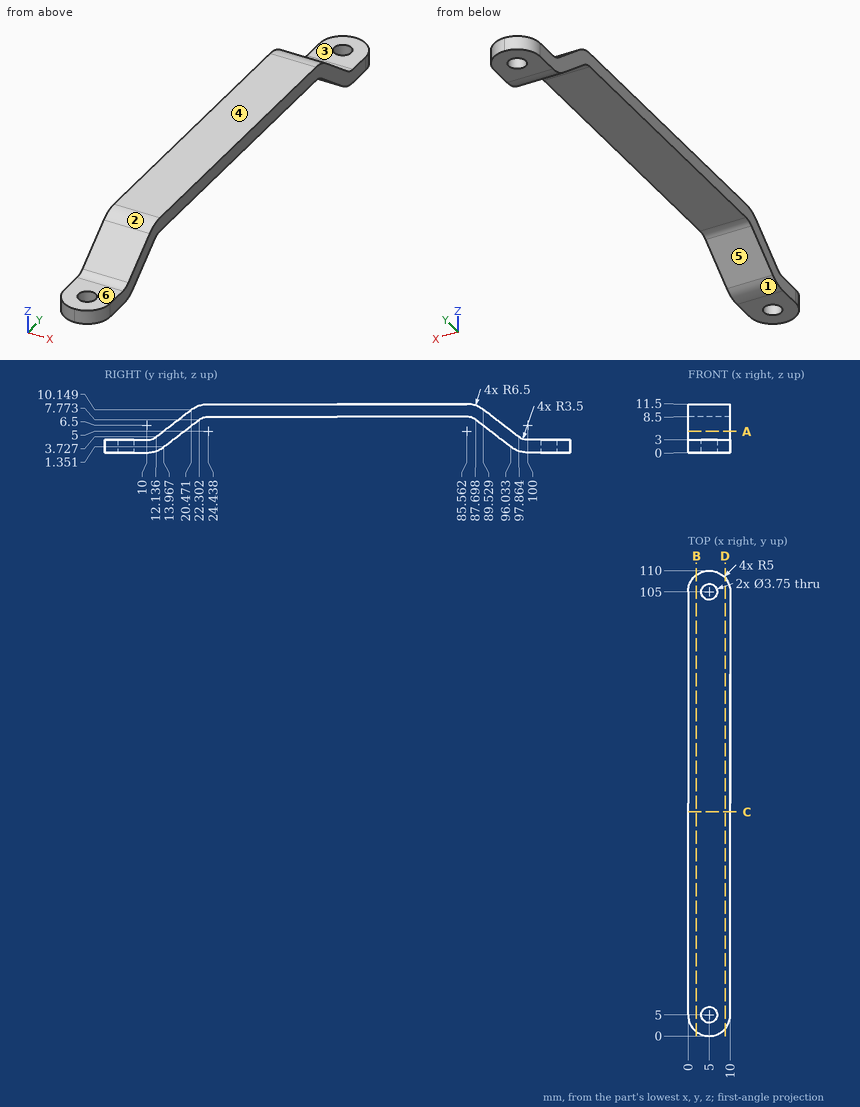
Check sheet for the drawn part. Datum: minimum x, y, z corner. Units: mm. A direction names the side the tool comes from. Round coordinates to 2 decimals unless told otherwise and drop trailing zeros. Order: outer loops, then holes, each group sorted by start corner. A loop starts at its lowest first (then second) coordinate and runs counter-clockwise, first axis right, second up. Notation, with made-up numbers: (79, 63.25) - (102, 63.25) arc R26 ccw to (102, 92.25) - close; hole circle Ø4 at (40, 0.5). An arc over 180 degrees is marked (long way). Use a Markdown table: item, result. Add a question column.
(1) Tool access check on the marked faces 4, 5 and 6. Record the directions out of +Z, -Z, +X, -X, +Y, -Y that give a thin tool (end or side, any length) a straight path to the whole face; none if there is none.
(2) Release check for a two-part mould opening along Y. For the marked faces 1, 2 and 3 record: pulls with the +Y half, pulls with the -Y half, needs draft (parallel to the pull), parting line crosses it, or undercut.
(3) Sectioned sample at C-C, the plane y = 53. Enter the section's corners in (x, z).
(4) Sectioned sample at D-D, the plane x = 8.75. Enter the section's corners in (y, z), and give its area (3 significant figures).
(5) Depth check by flat-ended pin: pin 1 (3 mm diameter, centred on x = 6, z = 10.5, fed in from +Y); pin 2 (5 mm diameter, centred on x = 6, y = 41, fed in from -Z); pin 3 (3.5 mm diameter, centred on x = 5, y = 105, fed in from +Z); pin 4 (5 mm diameter, centred on x = 7.5, y = 5, fed in from +Z). Enter the tip coordinate at first touch or a pass-through.
(6) Sectioned sample at A-A, the plane z = 5. Enter the section's corners in (x, y).
(7) Sectioned sample at B-B, the plane x = 2. Enter the section's corners in (y, z).
(8) Material ranges on line 1 along Y through (x, z) = (5, 1.75) (1 decimal); line 2 along Y through (x, z) = (5, 1.6) (1 decimal); line 3 along X through (y, z) = (105, 1.4) (1 decimal), recorded low to high. Write a range as [from, to].
Answers below:
| question | item | result |
|---|---|---|
| 1 | face 4 | +Z, +X, -X, +Y, -Y |
| 1 | face 5 | -Z, +X, -X |
| 1 | face 6 | +Z, +X, -X, -Y |
| 2 | face 1 | undercut |
| 2 | face 2 | pulls with the -Y half |
| 2 | face 3 | needs draft |
| 3 | outline | (0, 8.5) - (10, 8.5) - (10, 11.5) - (0, 11.5) - close |
| 4 | outline | (1.69, 0) - (10, 0) arc R6.5 ccw to (13.97, 1.35) - (22.3, 7.77) arc R3.5 cw to (24.44, 8.5) - (85.56, 8.5) arc R3.5 cw to (87.7, 7.77) - (96.03, 1.35) arc R6.5 ccw to (100, 0) - (108.31, 0) - (108.31, 3) - (100, 3) arc R3.5 cw to (97.86, 3.73) - (89.53, 10.15) arc R6.5 ccw to (85.56, 11.5) - (24.44, 11.5) arc R6.5 ccw to (20.47, 10.15) - (12.14, 3.73) arc R3.5 cw to (10, 3) - (1.69, 3) - close |
| 4 | area | 336 mm² |
| 5 | pin 1 | y = 91.02 |
| 5 | pin 2 | z = 8.5 |
| 5 | pin 3 | through |
| 5 | pin 4 | z = 3 |
| 6 | outline | (0, 13.79) - (10, 13.79) - (10, 18.7) - (0, 18.7) - close; (0, 91.3) - (10, 91.3) - (10, 96.21) - (0, 96.21) - close |
| 7 | outline | (1, 0) - (10, 0) arc R6.5 ccw to (13.97, 1.35) - (22.3, 7.77) arc R3.5 cw to (24.44, 8.5) - (85.56, 8.5) arc R3.5 cw to (87.7, 7.77) - (96.03, 1.35) arc R6.5 ccw to (100, 0) - (109, 0) - (109, 3) - (100, 3) arc R3.5 cw to (97.86, 3.73) - (89.53, 10.15) arc R6.5 ccw to (85.56, 11.5) - (24.44, 11.5) arc R6.5 ccw to (20.47, 10.15) - (12.14, 3.73) arc R3.5 cw to (10, 3) - (1, 3) - close |
| 8 | line 1 | [0, 3.1], [6.9, 14.5], [95.5, 103.1], [106.9, 110] |
| 8 | line 2 | [0, 3.1], [6.9, 14.3], [95.7, 103.1], [106.9, 110] |
| 8 | line 3 | [0, 3.1], [6.9, 10] |
